Here's how the part is built. I have some questions about the finished solid (model axes, mm). Round coordinates to 2 decimals unless told otherwise and drop trailing zeros. Write each loop counter-clockwise with the first axis right and the second up, starting at its lowest first coordinate (ties: lowest second). Pieces come first, ordered by that corner, then holes. Notation, with made-up numbers: (36, 50) -> (48, 50) arc R18 ccw to (48, 61) -> close; hole circle Ø7 at (-29, 17.25). An arc over 180 degrees is marked (long way). Answer as CSV lines item,"result".
Autodesk Inventor part; units mm, degrees
ref_plane "YZ Plane" through (0, 0, 0) normal (1, 0, 0) x (0, 1, 0)
ref_plane "XZ Plane" through (0, 0, 0) normal (0, 1, 0) x (-1, 0, 0)
ref_plane "XY Plane" through (0, 0, 0) normal (0, 0, 1) x (1, 0, 0)
sketch "Sketch1" plane through (0, 0, 0) normal (0, 1, 0) x (-1, 0, 0)
  line L0 (0, 0) -> (-482.6, 0)
  line L1 (-482.6, 0) -> (-482.6, -889)
  line L2 (-482.6, -889) -> (0, -889)
  line L3 (0, -889) -> (0, 0)
  line L4 (0, -889) -> (-25.4, -889)
  line L5 (-25.4, -889) -> (-25.4, -806.45)
  line L6 (-25.4, -806.45) -> (0, -806.45)
  line L7 (0, -806.45) -> (0, -889)
  line L8 (-25.4, -889) -> (-57.15, -889)
  line L9 (-57.15, -889) -> (-57.15, -863.6)
  line L10 (-57.15, -863.6) -> (-25.4, -863.6)
  line L11 (-25.4, -863.6) -> (-25.4, -889)
  line L12 (-241.3, -889) -> (-241.3, -324.207) construction
  line L13 (0, -444.5) -> (-482.6, -444.5) construction
  line L14 (-457.2, -889) -> (-457.2, -806.45)
  line L15 (-457.2, -806.45) -> (-482.6, -806.45)
  line L16 (-425.45, -889) -> (-425.45, -863.6)
  line L17 (-425.45, -863.6) -> (-457.2, -863.6)
  line L18 (-25.4, 0) -> (-25.4, -82.55)
  line L19 (-25.4, -82.55) -> (0, -82.55)
  line L20 (-57.15, 0) -> (-57.15, -25.4)
  line L21 (-57.15, -25.4) -> (-25.4, -25.4)
  line L22 (-457.2, -82.55) -> (-482.6, -82.55)
  line L23 (-457.2, 0) -> (-457.2, -82.55)
  line L24 (-425.45, -25.4) -> (-457.2, -25.4)
  line L25 (-425.45, 0) -> (-425.45, -25.4)
  point P0 (-482.6, -82.55)
  point P1 (-482.6, -806.45)
  point P2 (0, -806.45)
  point P3 (0, -82.55)
  point P4 (-457.2, -25.4)
  dimension "d0" = 482.6
  dimension "d1" = 889
  dimension "d2" = 25.4
  dimension "d3" = 82.55
  dimension "d4" = 31.75
  dimension "d5" = 25.4
extrude "Extrusion1" add sketch "Sketch1" along normal blind 6.35 contours L3 L6 L5 L10 L9 L2 L16 L17 L14 L15 L1 L22 L23 L24 L25 L0 L20 L21 L18 L19
properties part number "Robot bottom" material "Polycarbonate, Smoke"
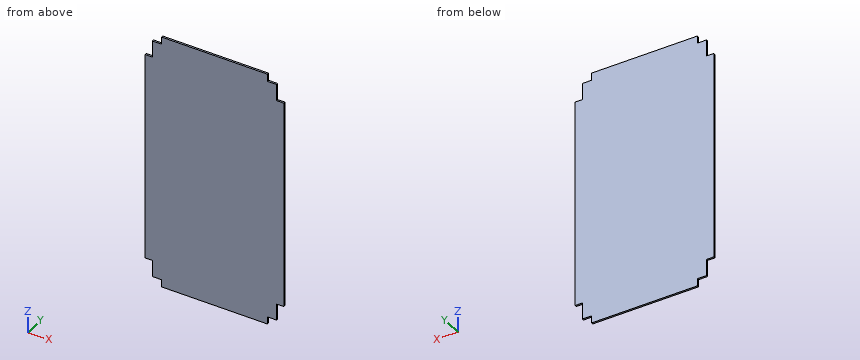
1. Suppose I cut it at A-A on y = 5.25. Please give me the cut outline in (x, z), and give its area (3 significant figures).
Numbers:
outline,"(0, -806.45) -> (25.4, -806.45) -> (25.4, -863.6) -> (57.15, -863.6) -> (57.15, -889) -> (425.45, -889) -> (425.45, -863.6) -> (457.2, -863.6) -> (457.2, -806.45) -> (482.6, -806.45) -> (482.6, -82.55) -> (457.2, -82.55) -> (457.2, -25.4) -> (425.45, -25.4) -> (425.45, 0) -> (57.15, 0) -> (57.15, -25.4) -> (25.4, -25.4) -> (25.4, -82.55) -> (0, -82.55) -> close"
area,"417,000 mm^2"
2. If I drill on line 1 (Z direction, x = 447, y = 5); line 2 (X direction, y = 4, z = -71), over which ranges is the centre line in solid material (lowest first)?
Numbers:
line 1,"z = -863.6 to -25.4"
line 2,"x = 25.4 to 457.2"
3. For pin 1 Ø1.9 at (y, z) = (2.5, -837.5) entering from +X; pin 2 Ø1.9 at (y, z) = (4, -842) entering from -X; pin 3 Ø3 at (x, y) = (39.5, 2) entering from -Z, each with a flat end and sliding along its axis, tell me the tip position at first contact or that it passes through.
Numbers:
pin 1,"stops at x = 457.2"
pin 2,"stops at x = 25.4"
pin 3,"stops at z = -863.6"
